from build123d import *

# Parameters (mm, degrees)
SKETCH1_R           = 1.651
BOSS_EXTRUDE1_DEPTH = 3.175
CUT_EXTRUDE1_START  = -3.175
CUT_EXTRUDE1_DEPTH  = 3.175


with BuildPart() as part:
    # Sketch1 → Boss-Extrude1 (new body)
    with BuildSketch(Plane(origin=(0, 0, 0), x_dir=(1, 0, 0), z_dir=(0, 1, 0))):
        with BuildLine():
            Line((-73.916912814, 12.7), (-73.916912814, -12.7))
            ThreePointArc((-73.916912814, -12.7), (-67.281551776, -33.138991997), (-55.122759171, -50.857461806))
            Line((-55.122759171, -50.857461806), (55.122759171, -50.857461806))
            ThreePointArc((55.122759171, -50.857461806), (61.833234068, -42.445861574), (67.270928268, -33.160552015))
            ThreePointArc((67.270928268, -33.160552015), (47.932265908, 0), (67.270928268, 33.160552015))
            ThreePointArc((67.270928268, 33.160552015), (61.833234068, 42.445861574), (55.122759171, 50.857461806))
            Line((55.122759171, 50.857461806), (-55.122759171, 50.857461806))
            ThreePointArc((-55.122759171, 50.857461806), (-67.281551776, 33.138991997), (-73.916912814, 12.7))
        make_face()
        with Locations(Location((0, -12.757461806, 0), (0, 0, 270))):
            Circle(SKETCH1_R, mode=Mode.SUBTRACT)
        with Locations(Location((0, -25.457461806, 0), (0, 0, 270))):
            Circle(SKETCH1_R, mode=Mode.SUBTRACT)
        with Locations(Location((31.75, -44.507461806, 0), (0, 0, 270))):
            Circle(SKETCH1_R, mode=Mode.SUBTRACT)
        with Locations(Location((-31.75, -44.507461806, 0), (0, 0, 270))):
            Circle(SKETCH1_R, mode=Mode.SUBTRACT)
        with Locations(Location((-52.26766059, 44.507461806, 0), (0, 0, 270))):
            Circle(SKETCH1_R, mode=Mode.SUBTRACT)
        with Locations(Location((-52.26766059, -44.507461806, 0), (0, 0, 270))):
            Circle(SKETCH1_R, mode=Mode.SUBTRACT)
        with Locations(Location((-31.75, 44.507461806, 0), (0, 0, 270))):
            Circle(SKETCH1_R, mode=Mode.SUBTRACT)
        with Locations(Location((31.75, 44.507461806, 0), (0, 0, 270))):
            Circle(SKETCH1_R, mode=Mode.SUBTRACT)
        with Locations(Location((0, 25.457461806, 0), (0, 0, 90))):
            Circle(SKETCH1_R, mode=Mode.SUBTRACT)
        with Locations(Location((0, 12.757461806, 0), (0, 0, 90))):
            Circle(SKETCH1_R, mode=Mode.SUBTRACT)
    extrude(amount=BOSS_EXTRUDE1_DEPTH)

    # Sketch2 → Cut-Extrude1 (cut)
    with BuildSketch(Plane(origin=(0, 3.175, 0), x_dir=(1, 0, 0), z_dir=(0, 1, 0)).offset(CUT_EXTRUDE1_START)):
        with BuildLine():
            Line((38.1, -50.857461806), (38.1, -38.157461806))
            Line((38.1, -38.157461806), (16.550455454, -38.157461806))
            Line((16.550455454, -38.157461806), (16.550455454, 38.157461806))
            Line((16.550455454, 38.157461806), (38.1, 38.157461806))
            Line((38.1, 38.157461806), (38.1, 50.857461806))
            Line((38.1, 50.857461806), (55.122759171, 50.857461806))
            ThreePointArc((55.122759171, 50.857461806), (61.833234068, 42.445861574), (67.270928268, 33.160552015))
            ThreePointArc((67.270928268, 33.160552015), (47.932265908, 0), (67.270928268, -33.160552015))
            ThreePointArc((67.270928268, -33.160552015), (61.833234068, -42.445861574), (55.122759171, -50.857461806))
            Line((55.122759171, -50.857461806), (38.1, -50.857461806))
        make_face()
        with BuildLine():
            Line((-64.601780161, 38.1), (-11.686912814, 38.1))
            Line((-11.686912814, 38.1), (-11.686912814, -38.1))
            Line((-11.686912814, -38.1), (-64.601780161, -38.1))
            ThreePointArc((-64.601780161, -38.1), (-70.414111341, -25.823495582), (-73.916912814, -12.7))
            Line((-73.916912814, -12.7), (-73.916912814, 12.7))
            ThreePointArc((-73.916912814, 12.7), (-70.414111341, 25.823495582), (-64.601780161, 38.1))
        make_face()
    extrude(amount=CUT_EXTRUDE1_DEPTH, mode=Mode.SUBTRACT)


solid = part.part
Read the model definition and answer for the solid it produces. Units are mm, in the model's axes. A direction names the side the tool comes from. Round coordinates to 2 decimals unless told otherwise and drop trailing zeros. Write each loop counter-clockwise with the first axis right and the second up, starting at its lowest first coordinate (ties: lowest second). Pieces come first, ordered by that corner, then holes.
1. The part is cut by section D-D, the plane z = 13. Determine the outline of the cut face in (x, y) (3 decimals), then the cut area to 3 significant figures.
2. Given pin 1 Ø1 at (y, z) = (1.5, -19) entering from -X, flat-ended and moving along its own axis, determine where the tip first touches the part or whether it passes through.
3. Which of the six approach directions +Z, -Z, +X, -X, +Y, -Y give full straight-line access (tool end or side, diameter ignored) to faces 1 (the face through (0.073, 1.565, 11.108)), 2 (the face through (-39, 2, -38.1)), 3 (the face through (27, 2, -38.157))?
4. The part is cut by section B-B, the plane x = 0. Determine the outline of the cut face in (y, z) (3 decimals).
5. Straight lines are drawn through the part: L1, parallel to Z at x = 24, y = 1.4; L2, parallel to Z at x = -21, y = 2; L3, parallel to X at y = 1.35, z = -26. For each, find the intervals that lie inside material, in ascending order.
6. Determine the mould class of faces 4 (the face through (-0.073, 1.565, -11.108)), 5 (the face through (-9, 2, 50.857)), 6 (the face through (-6, 0, 0)) for opening direction Z: pulls with the +Z half, pulls with the -Z half, needs draft (parallel to the pull), parting line crosses it, or undercut.
7. The part is cut by section C-C, the plane y = 1.1. State how many separate pieces and enclosed holes the cut face has, then the cut area to 3 significant figures.
8. The part is cut by section A-A, the plane x = 28.5. Determine the outline of the cut face in (y, z) (3 decimals).
Values:
1. outline: (-11.687, 0) - (-1.633, 0) - (-1.633, 3.175) - (-11.687, 3.175) - close; (1.633, 0) - (16.55, 0) - (16.55, 3.175) - (1.633, 3.175) - close
1. area: 79.3 mm2
2. pin 1: stops at x = -11.69
3. face 1: +Y, -Y
3. face 2: -X, +Y, -Y
3. face 3: +X, +Y, -Y
4. outline: (0, -50.857) - (3.175, -50.857) - (3.175, -27.108) - (0, -27.108) - close; (0, -23.806) - (3.175, -23.806) - (3.175, -14.408) - (0, -14.408) - close; (0, -11.106) - (3.175, -11.106) - (3.175, 11.106) - (0, 11.106) - close; (0, 14.408) - (3.175, 14.408) - (3.175, 23.806) - (0, 23.806) - close; (0, 27.108) - (3.175, 27.108) - (3.175, 50.857) - (0, 50.857) - close
5. L1: z = -50.86 to -38.16, 38.16 to 50.86
5. L2: z = -50.86 to -38.1, 38.1 to 50.86
5. L3: x = -11.69 to -1.56, 1.56 to 16.55
6. face 4: undercut
6. face 5: pulls with the +Z half
6. face 6: needs draft
7. separate pieces: 1
7. enclosed holes: 10
7. area: 4,570 mm2
8. outline: (0, -50.857) - (3.175, -50.857) - (3.175, -38.157) - (0, -38.157) - close; (0, 38.157) - (3.175, 38.157) - (3.175, 50.857) - (0, 50.857) - close
